Could you check a few things on this drawing? It's one solid part, dimensions in mm from its lowest x, y, z. Round coordinates to 2 decimals unless told otherwise and drop trailing zeros. Loops run counter-clockwise (first coordinate to the right, second up) from the corner with the lowest first, then second, coordinate; pieces in that order, holes last. Notation, with made-up numbers: (81, 40.25) -> (105, 40.25) arc R12 cw to (105, 44.25) -> close; hole circle Ø5 at (-30.5, 47). An arc over 180 degrees is marked (long way). Put each result on its own line as item: value. Start each with the question number.
1. I'm going to push flat-ended pins straight in: P1, Ø0.5, axis at x = 31, y = 2, coming from the +Z side (1 decimal); P2, Ø1, axis at y = 2, z = 15, coming from the +X side. Where does each tip first touch, or does it pass through?
2. Imagine slicing it at B-B, the plane y = 1.9. Please give me the cut outline in (x, z) (1 decimal).
3. I need wall thicknesses on line 1 (X direction, y = 2.3, z = 13.25); line 2 (Z direction, x = 51, y = 2) (1 decimal); line 3 (Y direction, x = 5.5, z = 1). Which ranges of each line are inside material? Lowest first, please. Write a range as [from, to].
4. Imagine slicing it at A-A, the plane x = 22.5. Please give me the cut outline in (y, z) (1 decimal), and give its area (3 significant figures).
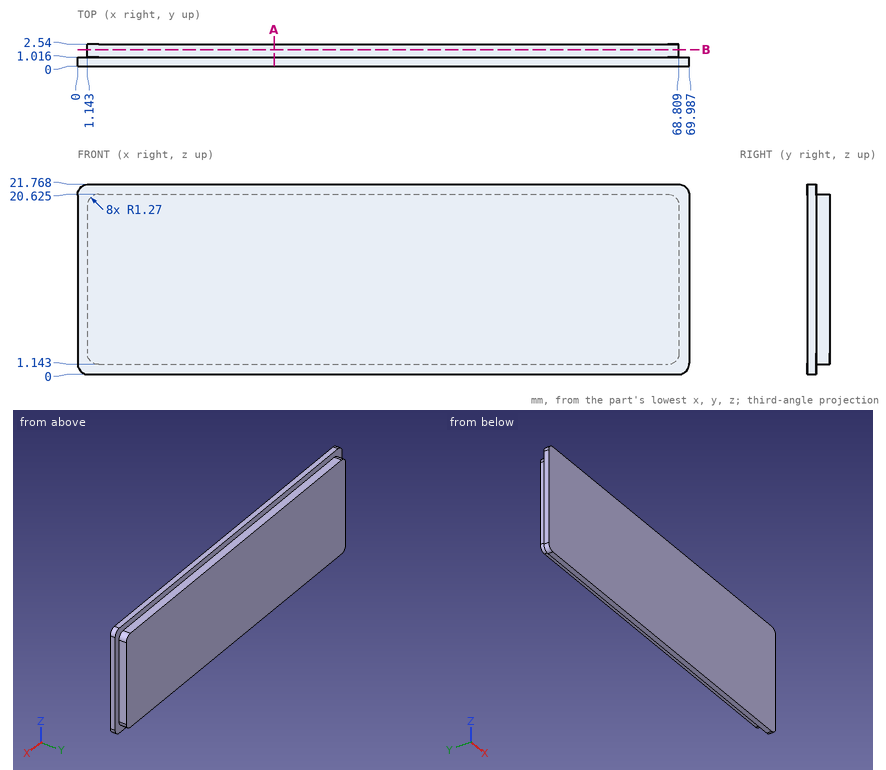
Entries:
1. P1: z = 20.6
1. P2: x = 68.81
2. outline: (1.1, 2.4) arc R1.3 ccw to (2.4, 1.1) -> (67.5, 1.1) arc R1.3 ccw to (68.8, 2.4) -> (68.8, 19.4) arc R1.3 ccw to (67.5, 20.6) -> (2.4, 20.6) arc R1.3 ccw to (1.1, 19.4) -> close
3. line 1: [1.14, 68.81]
3. line 2: [1.1, 20.6]
3. line 3: [0, 1.02]
4. outline: (0, 0) -> (1, 0) -> (1, 1.1) -> (2.5, 1.1) -> (2.5, 20.6) -> (1, 20.6) -> (1, 21.8) -> (0, 21.8) -> close
4. area: 51.8 mm^2
